Answer from the drawing. Dimensions are ordinates in mm from the lowest x, y and z of the part. A direction names the side the tool comes from. Give positions to 0.01 mm unless a question says otherwise; leave off trailing zeros. Loops run counter-clockwise (first coordinate to the right, second up) from the corner with the lowest first, then second, coordinate; pieces in that order, holes last.
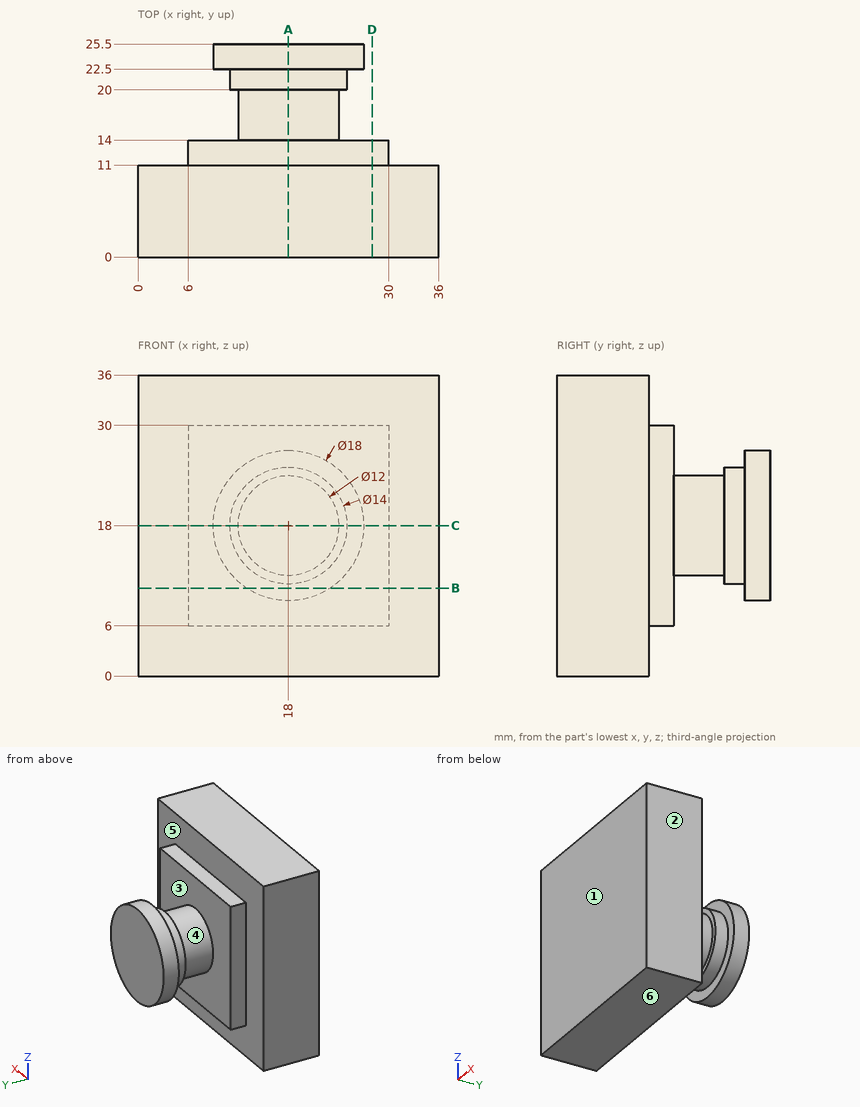
Item 1: For the marked faces 4, 5 and 6, determine the directions among +Z, -Z, +X, -X, +Y, -Y from which every point of the face is accessible in a straight line to the end or side of a thin tool.
Item 2: Flat-ended cylindrical pins translate along their axes: pin 1 Ø1 at (x, y) = (23.5, 22.5) entering from -Z; pin 2 Ø1 at (x, z) = (17, 27) entering from +Y; pin 3 Ø1.5 at (x, z) = (30.5, 15.5) entering from +Y; pin 4 Ø6 at (y, z) = (19, 21.5) entering from -X. Find the tip coordinate at first contact, or state that the pin passes through.
Item 3: Find section C-C, the plane z = 18. Write down the section's boundary in (x, y), plus the area to 3 significant figures.
Item 4: Find section D-D, the plane x = 28. Write down the section's boundary in (y, z), plus the area to 3 significant figures.
Item 5: Determine the mould class of the marked faces 1, 2 and 3 for opening direction Y: released by +Y, released by -Y, zero draft, split by the parting line, or undercut.
Item 6: Find section B-B, the plane z = 10.5. Write down the section's boundary in (x, y), plus the area to 3 significant figures.
Item 7: Consider line 1 (Y direction, x = 20, z = 26); line 2 (Y direction, x = 3, z = 29); line 3 (X direction, y = 13.75, z = 7.5). Determine where each line is inside the solid, lowest interval first.
Item 8: Find section A-A, the plane x = 18. Write down the section's boundary in (y, z).
Ans:
1. face 4: none
1. face 5: +Y
1. face 6: -Z, +X, -X, +Y, -Y
2. pin 1: stops at z = 10.52
2. pin 2: stops at y = 25.5
2. pin 3: stops at y = 14
2. pin 4: stops at x = 11.03
3. outline: (0, 0) - (36, 0) - (36, 11) - (30, 11) - (30, 14) - (24, 14) - (24, 20) - (25, 20) - (25, 22.5) - (27, 22.5) - (27, 25.5) - (9, 25.5) - (9, 22.5) - (11, 22.5) - (11, 20) - (12, 20) - (12, 14) - (6, 14) - (6, 11) - (0, 11) - close
3. area: 629 mm2
4. outline: (0, 0) - (11, 0) - (11, 6) - (14, 6) - (14, 30) - (11, 30) - (11, 36) - (0, 36) - close
4. area: 468 mm2
5. face 1: released by -Y
5. face 2: zero draft
5. face 3: undercut
6. outline: (0, 0) - (36, 0) - (36, 11) - (30, 11) - (30, 14) - (6, 14) - (6, 11) - (0, 11) - close; (13.03, 22.5) - (22.97, 22.5) - (22.97, 25.5) - (13.03, 25.5) - close
6. area: 498 mm2
7. line 1: y = 0 to 14, 22.5 to 25.5
7. line 2: y = 0 to 11
7. line 3: x = 6 to 30
8. outline: (0, 0) - (11, 0) - (11, 6) - (14, 6) - (14, 12) - (20, 12) - (20, 11) - (22.5, 11) - (22.5, 9) - (25.5, 9) - (25.5, 27) - (22.5, 27) - (22.5, 25) - (20, 25) - (20, 24) - (14, 24) - (14, 30) - (11, 30) - (11, 36) - (0, 36) - close
